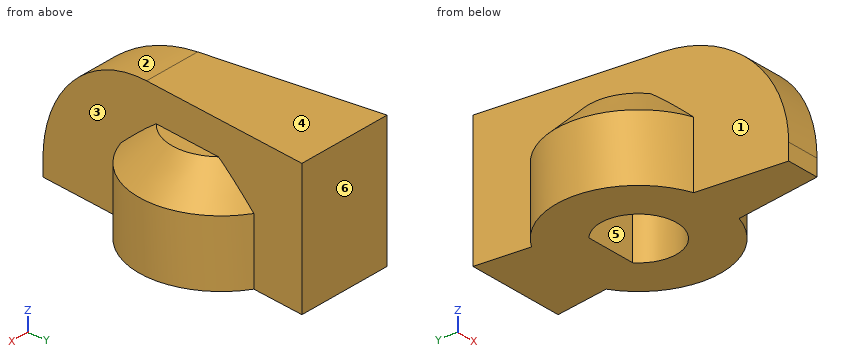
```python
from build123d import *

# Parameters (mm, degrees)
PAD_DEPTH    = 8
SKETCH001_R  = 5
PAD001_DEPTH = 6
POCKET_DEPTH = 5.5
PAD002_DEPTH = 1
CHAMFER_SIZE = 2
FILLET_R     = 7


with BuildPart() as part:
    # Sketch → Pad (new body)
    with BuildSketch(Plane.XY):
        Polygon((1, -10), (3, 7.5), (0, 7.5), (-3, 7.5), (-1, -10), (0, -10), align=None)
    extrude(amount=PAD_DEPTH)

    # Sketch001 (on Face2 of Pad) → Pad001 (join)
    with BuildSketch(Plane(origin=(0, 0, 0), x_dir=(1, 0, 0), z_dir=(0, 0, -1))):
        Circle(SKETCH001_R)
    extrude(amount=-PAD001_DEPTH)

    # Sketch002 (on Face9 of Pad001) → Pocket (cut)
    with BuildSketch(Plane(origin=(0, 0, 0), x_dir=(1, 0, 0), z_dir=(0, 0, -1))):
        with BuildLine():
            Line((-1.549193, -1.7), (1.549193, -1.7))
            ThreePointArc((1.549193, -1.7), (0, 2.3), (-1.549193, -1.7))
        make_face()
    extrude(amount=-POCKET_DEPTH, mode=Mode.SUBTRACT)

    # Sketch003 (on Face13 of Pocket) → Pad002 (join)
    with BuildSketch(Plane(origin=(0, 0, 5.5), x_dir=(1, 0, 0), z_dir=(0, 0, -1))):
        with BuildLine():
            Line((-2.286373, 0.25), (2.286373, 0.25))
            ThreePointArc((2.286373, -0.25), (2.313709, 0), (2.286373, 0.25))
            Line((-2.286373, -0.25), (2.286373, -0.25))
            ThreePointArc((-2.286373, 0.25), (-2.3, 0), (-2.286373, -0.25))
        make_face()
    extrude(amount=PAD002_DEPTH)

    # Chamfer
    chamfer_edges = [part.edges().sort_by_distance(p)[0] for p in [
        (4.062492, -2.914818, 6),
        (4.367186, 2.434685, 6),
        (-4.967663, -0.567733, 6),
    ]]
    chamfer(chamfer_edges, length=CHAMFER_SIZE)

    # Fillet
    fillet_edges = [part.edges().sort_by_distance(p)[0] for p in [
        (0, -10, 8),
    ]]
    fillet(fillet_edges, radius=FILLET_R)


solid = part.part
```
Verification items for the finished model (mm, model axes). Face numbers are marked on the shaded views. A direction names the side the tool comes from. Give positions to 0.01 mm unless a question says otherwise; leave off trailing zeros. Loops run counter-clockwise (first coordinate to the right, second up) from the corner with the lowest first, then second, coordinate; pieces in that order, holes last. Notation, with made-up numbers: M 49,80 L 58,80 A31 cw 58,114 Z; hole C 77.5,-21.5 d3. An arc over 180 degrees is marked long. One line per question, with ' | ' between items.
Item 1: Tool access check on the marked faces 1 and 2. Record the directions out of +Z, -Z, +X, -X, +Y, -Y that give a thin tool (end or side, any length) a straight path to the whole face; none if there is none.
Completed:
face 1: +Z, -X | face 2: +Z, +X, -X, -Y
Item 2: Section check B-B, the plane y = 0. Record the cut outline in (x, z).
Completed:
outline: M -5,0 L -2.3,0 L -2.3,4.5 L 2.3,4.5 L 2.3,0 L 5,0 L 5,4 L 3,6 L 2.14,6 L 2.14,8 L -2.14,8 L -2.14,6 L -3,6 L -5,4 Z
Item 3: Section check C-C, the plane x = 0. Record the cut outline in (y, z).
Completed:
outline: M -10,0 L -2.3,0 L -2.3,5.5 L -0.25,5.5 L -0.25,4.5 L 0.25,4.5 L 0.25,5.5 L 1.7,5.5 L 1.7,0 L 7.5,0 L 7.5,8 L -3,8 A7 ccw -10,1 Z
Item 4: Thickness scan on line 1 (X direction, y = 0, z = 2.6); line 2 (Y direction, x = 0, z = 1.45); line 3 (Y direction, x = 0, z = 2.8). Record the ranges inside material, lowest first. Write a range as [from, to].
Completed:
line 1: x = [-5, -2.3], [2.3, 5] | line 2: y = [-9.99, -2.3], [1.7, 7.5] | line 3: y = [-9.76, -2.3], [1.7, 7.5]
Item 5: Depth check by flat-ended pin: P1, Ø1.5, axis at x = 0.5, y = -8, coming from the +Z side; P2, Ø1.5, axis at x = 0.5, z = 4, coming from the -Y side; P3, Ø3, axis at x = -3.5, y = -5, coming from the +Z side. Enter the tip coordinate at first touch or a pass-through.
Completed:
P1: stops at z = 6.56 | P2: stops at y = -9.63 | P3: stops at z = 4.4
Item 6: Draft check along Y on the marked faces 3, 4, 5 and 6. Enter one of: +Y half, -Y half, draft (parallel to the pull), parting line (faces both ways), or undercut.
Completed:
face 3: undercut | face 4: draft | face 5: undercut | face 6: +Y half
Item 7: Section check D-D, the plane z = 0.75. Record the cut outline in (x, y), plus the area to 3 significant figures.
Completed:
outline: M -3,7.5 L -2.63,4.25 A5 ccw -1.6,-4.74 L -1,-10 L 1,-10 L 1.6,-4.74 A5 ccw 2.63,4.25 L 3,7.5 Z; hole M -1.55,1.7 A2.3 ccw long 1.55,1.7 Z | area: 91.9 mm^2
Item 8: Section check A-A, the plane z = 2.5. Record the cut outline in (x, y).
Completed:
outline: M -3,7.5 L -2.63,4.25 A5 ccw -1.6,-4.74 L -1.02,-9.84 L 1.02,-9.84 L 1.6,-4.74 A5 ccw 2.63,4.25 L 3,7.5 Z; hole M -1.55,1.7 A2.3 ccw long 1.55,1.7 Z
